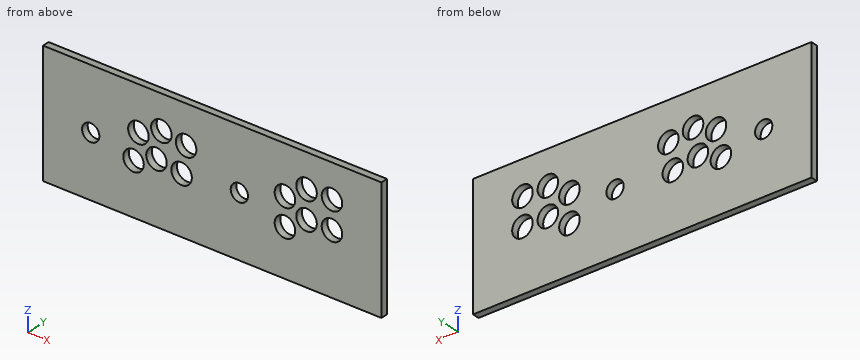
from build123d import *

# Parameters (mm, degrees)
F0_W     = 486
F0_H     = 175
F1_DEPTH = 10
F5_R     = 14.75
F5_R_2   = 12.4064380464
F7_DEPTH = 25
F3_R     = 14.75
F3_R_2   = 12.4065
F8_DEPTH = 25


# Not quite as in the source:
# - a feature names something its author has since deleted; it is built from what else it names


with BuildPart() as f1:
    # F0 (on Front) → F1 (new body)
    with BuildSketch(Plane.XZ):
        with Locations((243, 87.5)):
            Rectangle(F0_W, F0_H)
    extrude(amount=F1_DEPTH)

    # F5 (on face) → F7 (cut)
    with BuildSketch(Plane.XZ.offset(10)):
        with Locations((347.5, 106.75)):
            Circle(F5_R)
        with Locations((378.5, 127)):
            Circle(F5_R)
        with Locations((415, 127)):
            Circle(F5_R)
        with Locations((415, 87.5)):
            Circle(F5_R)
        with Locations((378.5, 87.5)):
            Circle(F5_R)
        with Locations((347.5, 67.25)):
            Circle(F5_R)
        with Locations((282, 87.5)):
            Circle(F5_R_2)
    extrude(amount=-F7_DEPTH, mode=Mode.SUBTRACT)

    # F3 (on face) → F8 (cut)
    with BuildSketch(Plane.XZ.offset(10)):
        with Locations((170, 126.3350188136)):
            Circle(F3_R)
        with Locations((205.5, 120.3350188136)):
            Circle(F3_R)
        with Locations((199, 81.8350188136)):
            Circle(F3_R)
        with Locations((163, 87.8350188136)):
            Circle(F3_R)
        with Locations((130, 73.8350188136)):
            Circle(F3_R)
        with Locations((137, 112.3350188136)):
            Circle(F3_R)
        with Locations((68.5, 87.5)):
            Circle(F3_R_2)
    extrude(amount=-F8_DEPTH, mode=Mode.SUBTRACT)


solid = f1.part
Could you check a few things on this model? Use its own coordinates, in mm. Coordinates: 2 decimals unless noted, no trailing zeros. Order: outer loops, then holes, each group sorted by start corner. A loop starts at its lowest first (then second) coordinate and runs counter-clockwise, first axis right, second up. Notation, with made-up numbers: (75.25, 34.25) -> (118.25, 34.25) arc R23 cw to (118.25, 53.25) -> close; hole circle Ø6 at (86.25, -27). An arc over 180 degrees is marked (long way). One line per item, written item: value. Start each with the question number.
1) Imagine slicing it at C-C on y = -1.75. Count the separate pieces of the cut face and the enclosed holes in it, plus the area to 3 significant figures.
2) Imagine slicing it at B-B on x = 68.5. List the corners of the cut face in (y, z) for me.
3) Imagine slicing it at D-D on x = 278. List the corners of the cut face in (y, z) for me.
4) Imagine slicing it at A-A on x = 415. List the corners of the cut face in (y, z) for me.
5) I'm going to push a flat-ended pin straight in: pin 1 (23.5 mm diameter, centred on x = 347.5, z = 67.25, fed in from -Y). Where does the tip first touch, or does it pass through?
6) If I drill on L1, parallel to Z at x = 347.5, y = -4.75; L2, parallel to Z at x = 378.5, y = -2.5; L3, parallel to X at y = -3.5, z = 124, over which ranges is the centre line in solid material (lowest first)? Write a range as [from, to].
Answer list:
1. separate pieces: 1
1. enclosed holes: 14
1. area: 75,900 mm2
2. outline: (-10, 0) -> (0, 0) -> (0, 75.09) -> (-10, 75.09) -> close; (-10, 99.91) -> (0, 99.91) -> (0, 175) -> (-10, 175) -> close
3. outline: (-10, 0) -> (0, 0) -> (0, 75.76) -> (-10, 75.76) -> close; (-10, 99.24) -> (0, 99.24) -> (0, 175) -> (-10, 175) -> close
4. outline: (-10, 0) -> (0, 0) -> (0, 72.75) -> (-10, 72.75) -> close; (-10, 102.25) -> (0, 102.25) -> (0, 112.25) -> (-10, 112.25) -> close; (-10, 141.75) -> (0, 141.75) -> (0, 175) -> (-10, 175) -> close
5. pin 1: passes through
6. L1: z = [0, 52.5], [82, 92], [121.5, 175]
6. L2: z = [0, 72.75], [102.25, 112.25], [141.75, 175]
6. L3: x = [0, 127.97], [146.03, 155.44], [184.56, 191.21], [219.79, 364.06], [392.94, 400.56], [429.44, 486]
